Answer from the drawing. Dimensions are ordinates in mm from the lowest x, y and z of the part. Give positions to 0.01 mm unless a question says otherwise; leave off trailing zeros. Write each loop counter-clockwise with the first axis right and the second up, starting at its lowest first coordinate (ties: lowest second). Pieces come first, ordered by that corner, then holes.
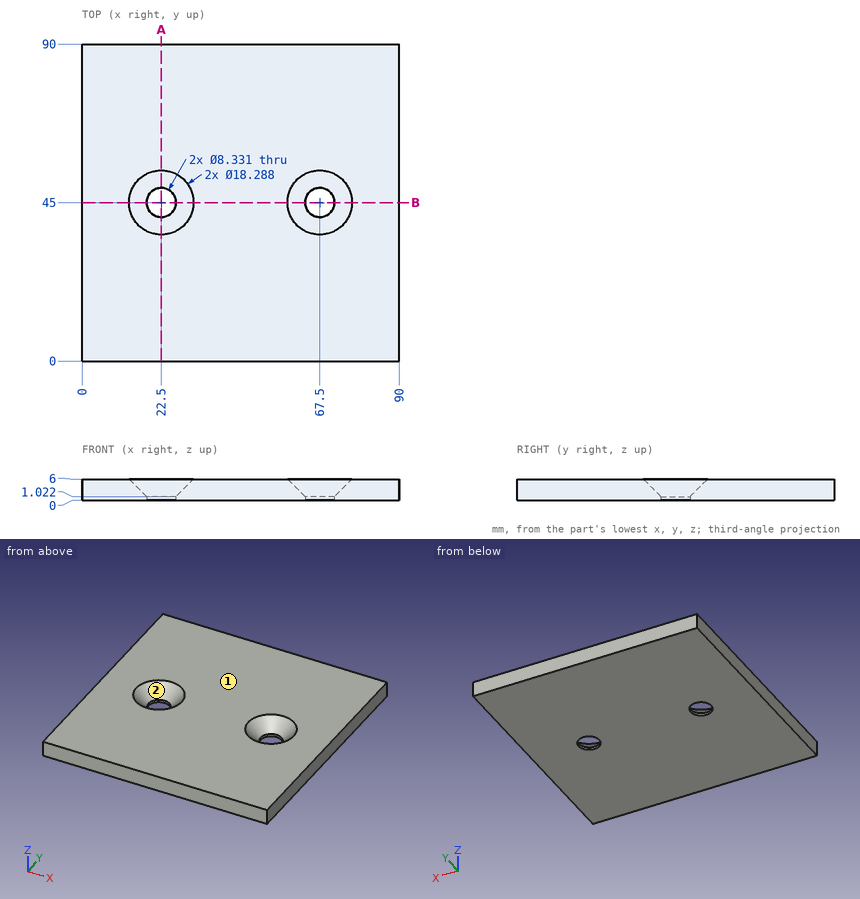
Item 1: Determine the mould class of the marked faces 1 and 2 for opening direction X: pulls with the +X half, pulls with the -X half, needs draft (parallel to the pull), parting line crosses it, or undercut.
Result set:
face 1: needs draft
face 2: undercut
Item 2: Each of these flat-tipped pins is pushed along its axis until it touches: pin 1 Ø11 at (x, y) = (22.5, 45) entering from +Z (1 decimal); pin 2 Ø5 at (x, y) = (67.5, 45) entering from +Z. Where does it stop, or does it pass through?
Result set:
pin 1: stops at z = 2.4
pin 2: passes through
Item 3: Section B-B (y = 45) is taken. Give the number of separate pieces and of enclosed holes in the cut face.
Result set:
separate pieces: 3
enclosed holes: 0
Item 4: Find the intervals of material crossed by line 1 along X through (y, z) = (45, 0.35) (1 decimal); line 2 along Y through (x, z) = (62, 3.75) (1 decimal); line 3 along Y through (x, z) = (65.5, 0.5) (1 decimal), in increasing order.
Result set:
line 1: x = 0 to 18.3, 26.7 to 63.3, 71.7 to 90
line 2: y = 0 to 40.8, 49.2 to 90
line 3: y = 0 to 41.3, 48.7 to 90
Item 5: Section A-A (x = 22.5) is taken. Write down the section's boundary in (y, z) (1 decimal).
Result set:
outline: (0, 0) - (40.8, 0) - (40.8, 1) - (35.9, 6) - (0, 6) - close; (49.2, 0) - (90, 0) - (90, 6) - (54.1, 6) - (49.2, 1) - close
